Verification items for the finished model (mm, model axes). Face numbers are marked on the shaded views. Coordinates: 2 decimals unless noted, no trailing zeros. Write each loop counter-clockwise with the first axis right and the second up, starting at its lowest first coordinate (ties: lowest second). Pieces come first, ordered by that corner, then holes. Notation, with made-up numbers: M -8.5,45 L 41.5,45 A24 ccw 41.5,79 Z; hole C 74.5,29.5 d4. An arc over 180 degrees is marked long. Answer in a Markdown table with one row per item.
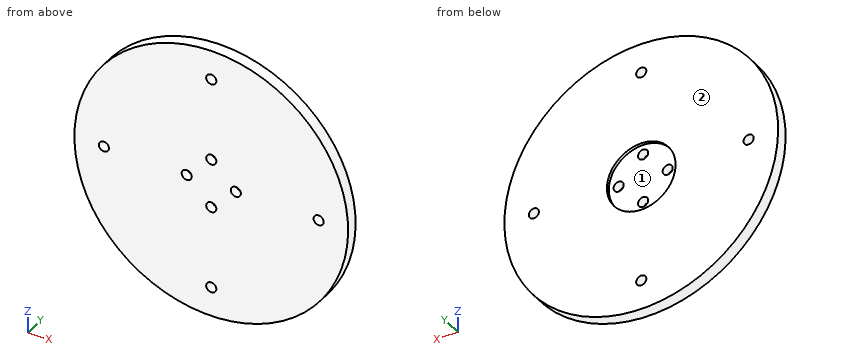
from build123d import *

# Parameters (mm, degrees)
SKETCH1_R           = 44.617697353
SKETCH1_R_2         = 1.65
BOSS_EXTRUDE1_DEPTH = 4
SKETCH2_R           = 11.2
CUT_EXTRUDE1_DEPTH  = 1


with BuildPart() as part:
    # Sketch1 → Boss-Extrude1 (new body)
    with BuildSketch(Plane(origin=(0, 0, 0), x_dir=(1, 0, 0), z_dir=(0, 1, 0))):
        with Locations(Location((0, 0, 0), (0, 0, 270))):
            Circle(SKETCH1_R)
        with Locations(Location((0, 8, 0), (0, 0, 270))):
            Circle(SKETCH1_R_2, mode=Mode.SUBTRACT)
        with Locations(Location((8, 0, 0), (0, 0, 270))):
            Circle(SKETCH1_R_2, mode=Mode.SUBTRACT)
        with Locations(Location((0, -8, 0), (0, 0, 270))):
            Circle(SKETCH1_R_2, mode=Mode.SUBTRACT)
        with Locations(Location((-8, 0, 0), (0, 0, 270))):
            Circle(SKETCH1_R_2, mode=Mode.SUBTRACT)
        with Locations(Location((0, 35, 0), (0, 0, 270))):
            Circle(SKETCH1_R_2, mode=Mode.SUBTRACT)
        with Locations(Location((35, 0, 0), (0, 0, 270))):
            Circle(SKETCH1_R_2, mode=Mode.SUBTRACT)
        with Locations(Location((0, -35, 0), (0, 0, 270))):
            Circle(SKETCH1_R_2, mode=Mode.SUBTRACT)
        with Locations(Location((-35, 0, 0), (0, 0, 270))):
            Circle(SKETCH1_R_2, mode=Mode.SUBTRACT)
    extrude(amount=BOSS_EXTRUDE1_DEPTH)

    # Sketch2 → Cut-Extrude1 (cut)
    with BuildSketch(Plane(origin=(0, 4, 0), x_dir=(1, 0, 0), z_dir=(0, 1, 0))):
        with Locations(Location((0, 0, 0), (0, 0, 270))):
            Circle(SKETCH2_R)
    extrude(amount=-CUT_EXTRUDE1_DEPTH, mode=Mode.SUBTRACT)


solid = part.part
1) Thickness scan on L1, parallel to X at y = 1.4, z = 0; L2, parallel to Z at x = -8, y = 2; L3, parallel to Y at x = 2, z = -1. Record the ranges inside material, lowest first. Write a range as [from, to].
Response values:
| item | result |
|---|---|
| L1 | x = [-44.62, -36.65], [-33.35, -9.65], [-6.35, 6.35], [9.65, 33.35], [36.65, 44.62] |
| L2 | z = [-43.89, -1.65], [1.65, 43.89] |
| L3 | y = [0, 3] |
2) Sectioned sample at D-D (z = 31). Record the cut outline in (x, y), then the cut area to 3 significant figures.
Response values:
| item | result |
|---|---|
| outline | M -32.09,0 L 32.09,0 L 32.09,4 L -32.09,4 Z |
| area | 257 mm² |
3) Sectioned sample at B-B (y = 1.85). Give the number of separate pieces and of enclosed holes in the cut face, then the cut area to 3 significant figures.
Response values:
| item | result |
|---|---|
| separate pieces | 1 |
| enclosed holes | 8 |
| area | 6,190 mm² |
4) Sectioned sample at C-C (z = 8). Record the cut outline in (x, y), then the cut area to 3 significant figures.
Response values:
| item | result |
|---|---|
| outline | M -43.89,0 L -1.65,0 L -1.65,3 L -7.84,3 L -7.84,4 L -43.89,4 Z; M 1.65,0 L 43.89,0 L 43.89,4 L 7.84,4 L 7.84,3 L 1.65,3 Z |
| area | 326 mm² |
5) Release check for a two-part mould opening along X. For the marked faces 1 and 2 record: +X half, -X half, draft (parallel to the pull), parting line (faces both ways), or undercut.
Response values:
| item | result |
|---|---|
| face 1 | undercut |
| face 2 | draft |
6) Depth check by flat-ended pin: pin 1 (5.5 mm diameter, centred on x = 0, z = -8, fed in from +Y); pin 2 (3 mm diameter, centred on x = -8, z = 0, fed in from +Y); pin 3 (1.5 mm diameter, centred on x = 30.5, y = 0.5, fed in from +Z). Enter the tip coordinate at first touch or a pass-through.
Response values:
| item | result |
|---|---|
| pin 1 | stops at y = 3 |
| pin 2 | passes through |
| pin 3 | stops at z = 33.25 |
7) Sectioned sample at A-A (x = 0). Record the cut outline in (y, z).
Response values:
| item | result |
|---|---|
| outline | M 0,-44.62 L 4,-44.62 L 4,-36.65 L 0,-36.65 Z; M 0,-33.35 L 4,-33.35 L 4,-11.2 L 3,-11.2 L 3,-9.65 L 0,-9.65 Z; M 0,-6.35 L 3,-6.35 L 3,6.35 L 0,6.35 Z; M 0,9.65 L 3,9.65 L 3,11.2 L 4,11.2 L 4,33.35 L 0,33.35 Z; M 0,36.65 L 4,36.65 L 4,44.62 L 0,44.62 Z |
